For this review, take the finished solid that the model builds, in its own axes (mm). A direction names the side the tool comes from. Coordinates: 2 decimals unless noted, no trailing zeros. Loops run counter-clockwise (first coordinate to the right, second up) from the corner with the lowest first, then second, coordinate; pieces in that order, holes last. Notation, with made-up numbers: (22.25, -19.75) - (38.25, -19.75) arc R25 ccw to (38.25, 15.25) - close; hole circle Ø9 at (-5, 45.25). An arc over 180 degrees is marked (long way). Use one line per item in the form item = value. Start each with the question number.
1. Add section A-A on x = -7.62. Give the boundary of the cut face in (y, z), and give its area (3 significant figures).
2. To check wall thickness, follow probe 1 along X at (y, z) = (-7.62, 6.75); probe 2 along Y at (x, z) = (3.5, 9). State the ranges of each line that lie inside material, in increasing order.
3. Machinability: for faces 1 (the face through (11, 2.84, 5)), 2 (the face through (-2.84, -11, 5)), 3 (the face through (2.84, 11, 5)), 4 (the face through (-11, 2.84, 5)), which of the approach directions +Z, -Z, +X, -X, +Y, -Y give a long, thin tool a straight path to every point of the face, cutting with its end or side? Answer none if there is none.
4. Add section C-C on z = 3. Give the boundary of the cut face in (x, y).
5. Draft analysis for pull direction Y (two halves, no side actions). For faces 5 (the face through (8, -12.7, 5)), 6 (the face through (-11, -2.84, 5)), 7 (the face through (-2.84, 11, 5)), 8 (the face through (8, 12.7, 5)), state which applies: +Y half, -Y half, draft (parallel to the pull), parting line (faces both ways), or undercut.
6. Add section D-D on y = 0. Give the boundary of the cut face in (x, z).
7. For pin 1 Ø1 at (x, z) = (-1, 4.5) entering from +Y, flat-tipped, find the tip position at first contact; note if it passes through.
```python
from build123d import *

# Parameters (mm, degrees)
F0_W            = 25.4
F0_H            = 25.4
F1_DEPTH        = 10.16
F2_R            = 3.81
F3_DEPTH        = 25.4
F3_COPIES_COUNT = 4
F5_DEPTH        = 25.4
F5_COPIES_COUNT = 4


# Not quite as in the source:
# - a pattern or mirror of a feature is missing from the dataset's text; its kind, count and spacing are read off the source's solid


with BuildPart() as f1:
    # F0 (on Top) → F1 (new body)
    with BuildSketch(Plane.XY):
        Rectangle(F0_W, F0_H)
    extrude(amount=F1_DEPTH)

    # F2 (on face) → F3 (cut)
    with BuildSketch(Plane.XY.offset(10.16)):
        with Locations((0, -7.62)):
            Circle(F2_R)
    f3 = extrude(amount=-F3_DEPTH, mode=Mode.SUBTRACT)

    # F3_copies: F3 ×4 about axis
    f3_copies_axis = Axis((0, 0, 0), (0, 0, 1))
    for i in range(1, F3_COPIES_COUNT):
        add(f3.rotate(f3_copies_axis, i * 360 / F3_COPIES_COUNT), mode=Mode.SUBTRACT)

    # F4 (on face) → F5 (cut)
    with BuildSketch(Plane.XY.offset(10.16)):
        with BuildLine():
            Line((-2.8398063314, -10.16), (-2.8398063314, -12.7))
            Line((-2.8398063314, -12.7), (2.8398063314, -12.7))
            Line((2.8398063314, -12.7), (2.8398063314, -10.16))
            ThreePointArc((2.8398063314, -10.16), (0, -11.43), (-2.8398063314, -10.16))
        make_face()
    f5 = extrude(amount=-F5_DEPTH, mode=Mode.SUBTRACT)

    # F5_copies: F5 ×4 about axis
    f5_copies_axis = Axis((0, 0, 0), (0, 0, 1))
    for i in range(1, F5_COPIES_COUNT):
        add(f5.rotate(f5_copies_axis, i * 360 / F5_COPIES_COUNT), mode=Mode.SUBTRACT)


solid = f1.part
```
Conclusion:
q1.outline = (-12.7, 0) - (-3.81, 0) - (-3.81, 10.16) - (-12.7, 10.16) - close; (3.81, 0) - (12.7, 0) - (12.7, 10.16) - (3.81, 10.16) - close
q1.area = 181 mm^2
q2.probe_1 = -12.7 to -3.81, 3.81 to 12.7
q2.probe_2 = -12.7 to -9.13, -6.11 to 6.11, 9.13 to 12.7
q3.face_1 = +Z, -Z, +X
q3.face_2 = +Z, -Z, -Y
q3.face_3 = +Z, -Z, +Y
q3.face_4 = +Z, -Z, -X
q4.outline = (-12.7, -12.7) - (-2.84, -12.7) - (-2.84, -10.16) arc R3.81 cw (long way) to (2.84, -10.16) - (2.84, -12.7) - (12.7, -12.7) - (12.7, -2.84) - (10.16, -2.84) arc R3.81 cw (long way) to (10.16, 2.84) - (12.7, 2.84) - (12.7, 12.7) - (2.84, 12.7) - (2.84, 10.16) arc R3.81 cw (long way) to (-2.84, 10.16) - (-2.84, 12.7) - (-12.7, 12.7) - (-12.7, 2.84) - (-10.16, 2.84) arc R3.81 cw (long way) to (-10.16, -2.84) - (-12.7, -2.84) - close
q5.face_5 = -Y half
q5.face_6 = undercut
q5.face_7 = draft
q5.face_8 = +Y half
q6.outline = (-3.81, 0) - (3.81, 0) - (3.81, 10.16) - (-3.81, 10.16) - close
q7.pin_1 = 4.12
